Model file for the job. Use its own axes, mm. A direction names the side the tool comes from. Round coordinates to 2 decimals unless told otherwise and drop trailing zeros. Loops run counter-clockwise (first coordinate to the right, second up) from the corner with the lowest first, then second, coordinate; pieces in that order, holes last. Notation, with made-up numbers: M 61,-36 L 66,-36 A7 ccw 66,-24 Z; hole C 36.5,16 d4. An arc over 180 degrees is marked long. Answer in a Markdown table with one row per item.
from build123d import *

# Parameters (mm, degrees)
BOSS_EXTRUDE1_DEPTH = 18
BOSS_EXTRUDE2_DEPTH = 18
SKETCH2_R           = 2.7
CUT_EXTRUDE1_DEPTH  = 60.970253183
SKETCH3_W           = 21
SKETCH3_H           = 6
CUT_EXTRUDE2_DEPTH  = 60.970253183
CUT_EXTRUDE5_DEPTH  = 60.970253183
SKETCH5_R           = 5
CUT_EXTRUDE4_DEPTH  = 4
FILLET1_R           = 4


with BuildPart() as part:
    # Sketch1 → Boss-Extrude1 (new body)
    with BuildSketch(Plane(origin=(0, 0, 0), x_dir=(1, 0, 0), z_dir=(0, 1, 0))):
        Polygon((37.602648402, 29.11), (37.602648402, 11), (16.67, 0), (0, 0), (0, 9.35), (0, 15.35), (37.602648402, 35.11), align=None)
    extrude(amount=BOSS_EXTRUDE1_DEPTH)

    # Sketch6 → Boss-Extrude2 (add, through all)
    with BuildSketch(Plane(origin=(0, 18, 0), x_dir=(1, 0, 0), z_dir=(0, 1, 0))):
        Polygon((0, 0), (-8, 0), (-8, 19.146040792), (37.602648402, 43.11), (37.602648402, 35.11), (0, 15.35), align=None)
    extrude(amount=-BOSS_EXTRUDE2_DEPTH)

    # Sketch2 → Cut-Extrude1 (cut, through all)
    with BuildSketch(Plane(origin=(0, 18, 0), x_dir=(1, 0, 0), z_dir=(0, 1, 0))):
        with Locations(Location((4, 6, 0), (0, 0, 270))):
            Circle(SKETCH2_R)
        with Locations(Location((21.62, 9.06, 0), (0, 0, 270))):
            Circle(SKETCH2_R)
        with Locations(Location((27.62, 19.16, 0), (0, 0, 270))):
            Circle(SKETCH2_R)
    extrude(amount=-CUT_EXTRUDE1_DEPTH, mode=Mode.SUBTRACT)

    # Sketch3 → Cut-Extrude2 (cut, through all)
    with BuildSketch(Plane.XY):
        with Locations((27.102648402, 9)):
            Rectangle(SKETCH3_W, SKETCH3_H)
    extrude(amount=-CUT_EXTRUDE2_DEPTH, mode=Mode.SUBTRACT)

    # Sketch4 → Cut-Extrude5 (cut, through all)
    with BuildSketch(Plane(origin=(0, 18, 0), x_dir=(1, 0, 0), z_dir=(0, 1, 0))):
        Polygon((-8, 0), (-8, 1), (-7, 0), (-6, 1), (-5, 0), (-4, 1), (-3, 0), (-2, 1), (-1, 0), (0, 1), (1, 0), (2, 1), (3, 0), (4, 1), (5, 0), (6, 1), (7, 0), (8, 1), (9, 0), (10, 1), (11, 0), (12, 1), (13, 0), (14, 1), (15, 0), (16, 1), (16.88632324, 0.11367676), (16.67, 0), (16.67, -0.2), (-8, -0.2), align=None)
    extrude(amount=-CUT_EXTRUDE5_DEPTH, mode=Mode.SUBTRACT)

    # Sketch5 → Cut-Extrude4 (cut)
    with BuildSketch(Plane.XZ):
        with Locations(Location((21.62, -9.06, 0), (0, 0, 270))):
            Circle(SKETCH5_R)
        with Locations(Location((27.62, -19.16, 0), (0, 0, 270))):
            Circle(SKETCH5_R)
    cut_extrude4 = extrude(amount=-CUT_EXTRUDE4_DEPTH, mode=Mode.SUBTRACT)

    # Mirror1: Cut-Extrude4 across plane
    add(cut_extrude4.mirror(Plane(origin=(0, 9, 0), x_dir=(0, 0, 1), z_dir=(0, -1, 0))), mode=Mode.SUBTRACT)

    # Fillet1
    fillet1_edges = [part.edges().sort_by_distance(p)[0] for p in [
        (37.602648402, 15, -11),
        (-8, 9, -19.146040792),
        (37.602648402, 3, -43.11),
        (37.602648402, 15, -43.11),
        (37.602648402, 3, -11),
    ]]
    fillet(fillet1_edges, radius=FILLET1_R)


solid = part.part
1. Saw through at B-B (z = -35). Write the cut outline in (x, y), and give its area (3 significant figures).
Verdict:
| item | result |
|---|---|
| outline | M 22.17,0 L 37.6,0 L 37.6,6 L 22.17,6 Z; M 22.17,12 L 37.6,12 L 37.6,18 L 22.17,18 Z |
| area | 185 mm² |
2. Wall check: probe 1 along Y at (x, z) = (27, -27); probe 2 along X at (y, z) = (17, -7.5) (3 decimals); probe 3 along X at (y, z) = (13.1, -9.06). Give the ranges that are in metal, low to high.
Verdict:
| item | result |
|---|---|
| probe 1 | y = 0 to 6, 12 to 18 |
| probe 2 | x = -8 to 1.755, 6.245 to 16.87, 26.37 to 30.942 |
| probe 3 | x = -8 to 18.92, 24.32 to 33.91 |
3. Mould opens along Z. For faces 4 (the flat face through (-8, 9, -9)), 5 (the flat face through (25, 4, -21)), 6 (the flat face through (15.5, 9.1, -0.5)), 7 (the flat face through (25, 14, -21)) say: +Z half, -Z half, draft (parallel to the pull), parting line (faces both ways), or undercut.
Verdict:
| item | result |
|---|---|
| face 4 | draft |
| face 5 | undercut |
| face 6 | +Z half |
| face 7 | undercut |
4. Saw through at D-D (z = -19.5). Write the cut outline in (x, y).
Verdict:
| item | result |
|---|---|
| outline | M -6.89,0 L 22.63,0 L 22.63,4 L 24.94,4 L 24.94,6 L 16.6,6 L 16.6,12 L 24.94,12 L 24.94,14 L 22.63,14 L 22.63,18 L -6.89,18 Z; M 30.3,4 L 32.61,4 L 32.61,0 L 37.6,0 L 37.6,6 L 30.3,6 Z; M 30.3,12 L 37.6,12 L 37.6,18 L 32.61,18 L 32.61,14 L 30.3,14 Z |
5. Saw through at A-A (x = 27.62). Write the cut outline in (y, z), and give its area (3 significant figures).
Verdict:
| item | result |
|---|---|
| outline | M 0,-37.86 L 6,-37.86 L 6,-21.86 L 4,-21.86 L 4,-24.16 L 0,-24.16 Z; M 0,-14.16 L 4,-14.16 L 4,-16.46 L 6,-16.46 L 6,-5.75 L 0,-5.75 Z; M 12,-37.86 L 18,-37.86 L 18,-24.16 L 14,-24.16 L 14,-21.86 L 12,-21.86 Z; M 12,-16.46 L 14,-16.46 L 14,-14.16 L 18,-14.16 L 18,-5.75 L 12,-5.75 Z |
| area | 284 mm² |
6. Tool access for faces 1 (the flat face through (-1.5, 9.1, -0.5)), 2 (the cylindrical face through (1.605, 9.126, -4.754)), 3 (the flat face through (16.603, 9, -16)): list every direction of +Z, -Z, +X, -X, +Y, -Y with a clear straight run to the whole face (end or side of a thin tool).
Verdict:
| item | result |
|---|---|
| face 1 | +Z, +Y, -Y |
| face 2 | +Y, -Y |
| face 3 | +Z, -Z, +X |
7. Pin check, flat tips, straight feed: pin 1 (6 mm diameter, centred on x = 15, y = 3.5, fed in from -Z); pin 2 (5 mm diameter, centred on x = 25.5, y = 15, fed in from +Z); pin 3 (10 mm diameter, centred on x = 32.5, y = 6.5, fed in from +Z). Stop position of each tip, or through.
Verdict:
| item | result |
|---|---|
| pin 1 | stops at z = -32.81 |
| pin 2 | stops at z = -3.33 |
| pin 3 | stops at z = -5.7 |
